For this review, take the finished solid that the model builds, in its own axes (mm). Give positions to 0.01 mm unless a question says otherwise; leave off trailing zeros. Write each loop counter-clockwise with the first axis right and the second up, starting at its lowest first coordinate (ties: lowest second). Pieces come first, ordered by that corner, then holes. Notation, with made-up numbers: (80.5, -13) -> (129.5, -13) arc R12 cw to (129.5, 1) -> close; hole circle Ø8 at (50, -17.5). An arc over 180 degrees is marked (long way). Return JSON: item names as keys, results as strings.
from build123d import *

# Parameters (mm, degrees)
BOSS_EXTRUDE1_DEPTH       = 6.35
SKETCH2_R                 = 92.71
CUT_EXTRUDE1_DEPTH        = 7.35
F_8_CLEARANCE_HOLE1_D     = 4.4958
F_8_CLEARANCE_HOLE1_DEPTH = 25.4
F_8_CLEARANCE_HOLE1_TIP   = 1.350674586


with BuildPart() as part:
    # Sketch1 → Boss-Extrude1 (new body)
    with BuildSketch(Plane(origin=(0, 0, 0), x_dir=(0, 0, -1), z_dir=(1, 0, 0))):
        Polygon((0, 0), (558.8, 0), (374.65, 325.68545203), (184.15, 325.68545203), align=None)
    extrude(amount=BOSS_EXTRUDE1_DEPTH)

    # Sketch2 → Cut-Extrude1 (cut, through all)
    with BuildSketch(Plane(origin=(6.35, 0, 0), x_dir=(0, 0, -1), z_dir=(1, 0, 0))):
        with Locations((279.4, 146.05)):
            Circle(SKETCH2_R)
    extrude(amount=-CUT_EXTRUDE1_DEPTH, mode=Mode.SUBTRACT)

    # #8 Clearance Hole1
    with Locations(Plane.ZY):
        with Locations((-336.55, 245.036703653), (-222.25, 245.036703653), (-165.1, 146.05), (-222.25, 47.063296347), (-336.55, 47.063296347), (-393.7, 146.05)):
            Hole(F_8_CLEARANCE_HOLE1_D / 2, depth=F_8_CLEARANCE_HOLE1_DEPTH)
            with Locations((0, 0, -(F_8_CLEARANCE_HOLE1_DEPTH + F_8_CLEARANCE_HOLE1_TIP / 2))):  # 118° drill point
                Cone(0, F_8_CLEARANCE_HOLE1_D / 2, F_8_CLEARANCE_HOLE1_TIP, mode=Mode.SUBTRACT)


solid = part.part
1. Add section D-D, the plane z = -454. State the section outline as (x, y) points, plus the area to 3 significant figures.
Results found:
{"outline": "(0, 0) -> (6.35, 0) -> (6.35, 185.35) -> (0, 185.35) -> close", "area": "1,180 mm²"}
2. The part is to be moulded in two halves that separate along Y. For faces 1 (the flat face through (6.35, 57, -338)), 2 (the flat face through (3.131, 160.563, -468.014)), 3 (the cylindrical face through (3.22, 208.71, -211.07)), say which applies: +Y half, -Y half, draft (parallel to the pull), parting line (faces both ways), or undercut.
Results found:
{"face 1": "draft", "face 2": "+Y half", "face 3": "undercut"}
3. To check wall thickness, follow probe 1 along Y at (x, z) = (2.75, -336.55); probe 2 along Y at (x, z) = (4.5, -279.4); probe 3 along Z at (x, y) = (0.5, 131). State the ranges of each line that lie inside material, in increasing order.
Results found:
{"probe 1": "y = 0 to 44.82, 49.31 to 73.05, 219.05 to 242.79, 247.28 to 325.69", "probe 2": "y = 0 to 53.34, 238.76 to 325.69", "probe 3": "z = -484.73 to -370.88, -187.92 to -74.07"}
4. Add section A-A, the plane z = -279.4. State the section outline as (x, y) points, plus the area to 3 significant figures.
Results found:
{"outline": "(0, 0) -> (6.35, 0) -> (6.35, 53.34) -> (0, 53.34) -> close; (0, 238.76) -> (6.35, 238.76) -> (6.35, 325.69) -> (0, 325.69) -> close", "area": "891 mm²"}
5. Add section B-B, the plane y = 119. State the section outline as (x, z) points, plus the area to 3 significant figures.
Results found:
{"outline": "(0, -491.51) -> (6.35, -491.51) -> (6.35, -368.08) -> (0, -368.08) -> close; (0, -190.72) -> (6.35, -190.72) -> (6.35, -67.29) -> (0, -67.29) -> close", "area": "1,570 mm²"}
6. Add section C-C, the plane x = 4. State the section outline as (y, z) points, plus the area to 3 significant figures.
Results found:
{"outline": "(0, -558.8) -> (325.69, -374.65) -> (325.69, -184.15) -> (0, 0) -> close; hole circle Ø4.5 at (47.06, -336.55); hole circle Ø4.5 at (47.06, -222.25); hole circle Ø185.42 at (146.05, -279.4); hole circle Ø4.5 at (146.05, -393.7); hole circle Ø4.5 at (146.05, -165.1); hole circle Ø4.5 at (245.04, -336.55); hole circle Ø4.5 at (245.04, -222.25)", "area": "94,900 mm²"}
